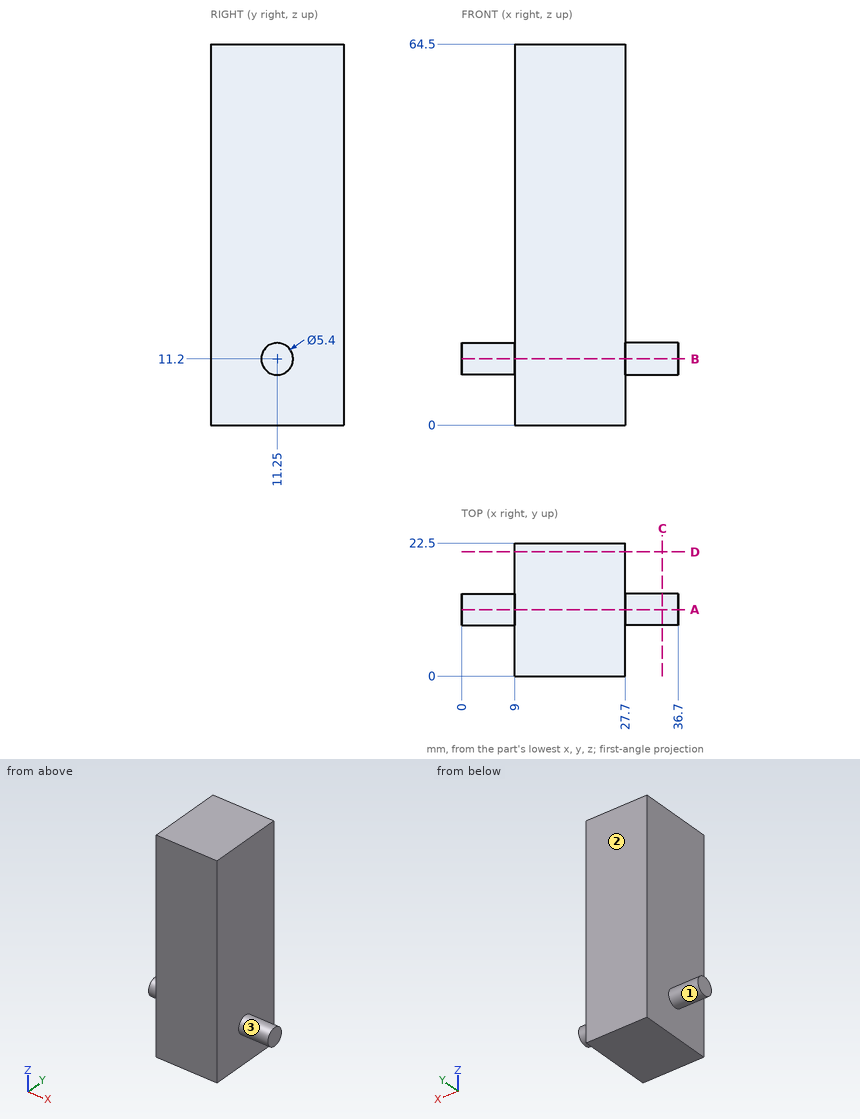
Design review of the part shown in the three views and the two pictorial views. Dimensions are in mm from the part's minimum x, y and z. A direction names the side the tool comes from. Round coordinates to 2 decimals unless told otherwise and drop trailing zeros. Loops run counter-clockwise (first coordinate to the right, second up) from the corner with the lowest first, then second, coordinate; pieces in that order, holes last. Notation, with made-up numbers: (80, 76.5) - (86, 76.5) arc R25 cw to (86, 107.5) - close; hole circle Ø1 at (60, 14). An arc over 180 degrees is marked (long way). Use CSV: the item, a comma, the result in double quotes.
(1) Machinability: for the marked faces 1, 2 and 3, which of the approach directions +Z, -Z, +X, -X, +Y, -Y give a long, thin tool a straight path to every point of the face, cutting with its end or side? Answer none if there is none.
Working result:
face 1,"-X"
face 2,"+Z, -Z, +X, -X, +Y"
face 3,"+X"
(2) Clearance check with flat-ended pins moving along their axes: P1, Ø2, axis at y = 18.5, z = 43, coming from the +X side; P2, Ø1, axis at y = 13.5, z = 48.5, coming from the -X side. State where each tip first meets the part, or that it passes through.
Working result:
P1,"stops at x = 27.7"
P2,"stops at x = 9"
(3) For line 1 (X direction, y = 6.75, z = 5); line 2 (Z direction, x = 8, y = 12.5), list the stretches that pass through material, from the lowest coordinate up.
Working result:
line 1,"x = 9 to 27.7"
line 2,"z = 8.81 to 13.59"
(4) Take a section at A-A, the plane y = 11.25. Give the boundary of the cut face in (x, z), plus the area to 3 significant figures.
Working result:
outline,"(0, 8.5) - (9, 8.5) - (9, 0) - (27.7, 0) - (27.7, 8.5) - (36.7, 8.5) - (36.7, 13.9) - (27.7, 13.9) - (27.7, 64.5) - (9, 64.5) - (9, 13.9) - (0, 13.9) - close"
area,"1,300 mm^2"
(5) Take a section at B-B, the plane z = 11.2. Give the boundary of the cut face in (x, y).
Working result:
outline,"(0, 8.55) - (9, 8.55) - (9, 0) - (27.7, 0) - (27.7, 8.55) - (36.7, 8.55) - (36.7, 13.95) - (27.7, 13.95) - (27.7, 22.5) - (9, 22.5) - (9, 13.95) - (0, 13.95) - close"
(6) Take a section at C-C, the plane x = 34. Give the boundary of the cut face in (y, z), plus the area to 3 significant figures.
Working result:
outline,"circle Ø5.4 at (11.25, 11.2)"
area,"22.9 mm^2"
(7) Take a section at D-D, the plane y = 21. Give the boundary of the cut face in (x, z), plus the area to 3 significant figures.
Working result:
outline,"(9, 0) - (27.7, 0) - (27.7, 64.5) - (9, 64.5) - close"
area,"1,210 mm^2"
